Check sheet for the modelled part. Datum: model origin and axes. Units: mm. A direction names the side the tool comes from. Round coordinates to 2 decimals unless told otherwise and drop trailing zeros. Write each loop counter-clockwise with the first axis right and the second up, starting at its lowest first coordinate (ties: lowest second). Pieces come first, ordered by that corner, then holes.
from build123d import *

# Parameters (mm, degrees)
BOSS_EXTRUDE1_DEPTH = 10
BOSS_EXTRUDE2_DEPTH = 10
SKETCH3_R           = 7.5
BOSS_EXTRUDE3_DEPTH = 145
SKETCH4_R           = 2.5
BOSS_EXTRUDE4_DEPTH = 145
SKETCH6_R           = 12.5
CUT_EXTRUDE1_DEPTH  = 165
SKETCH9_R           = 7.5
CUT_EXTRUDE2_DEPTH  = 25
SKETCH11_R          = 15
BOSS_EXTRUDE6_DEPTH = 20
SKETCH12_R          = 15
BOSS_EXTRUDE7_DEPTH = 20
SKETCH13_R          = 15
CUT_EXTRUDE6_DEPTH  = 25


with BuildPart() as part:
    # Sketch1 → Boss-Extrude1 (new body)
    with BuildSketch(Plane.XY):
        with BuildLine():
            Line((-265, 35), (265, 35))
            ThreePointArc((265, 35), (300, 0), (265, -35))
            Line((265, -35), (-265, -35))
            ThreePointArc((-265, -35), (-300, 0), (-265, 35))
        make_face()
    extrude(amount=BOSS_EXTRUDE1_DEPTH)



with BuildPart() as body_2:
    # Sketch2 → Boss-Extrude2 (new body)
    with BuildSketch(Plane.XY.offset(-100)):
        with BuildLine():
            Line((-265, 35), (265, 35))
            ThreePointArc((265, 35), (300, 0), (265, -35))
            Line((265, -35), (-265, -35))
            ThreePointArc((-265, -35), (-300, 0), (-265, 35))
        make_face()
    extrude(amount=-BOSS_EXTRUDE2_DEPTH)


with BuildPart() as part_1:
    add(part.part)

    add(body_2.part)  # Boss-Extrude3 merges body 2
    # Sketch3 → Boss-Extrude3 (add)
    with BuildSketch(Plane(origin=(0, 0, -110), x_dir=(-1, 0, 0), z_dir=(0, 0, -1))):
        Circle(SKETCH3_R)
    extrude(amount=-BOSS_EXTRUDE3_DEPTH)

    # Sketch4 → Boss-Extrude4 (add)
    with BuildSketch(Plane(origin=(0, 0, -110), x_dir=(-1, 0, 0), z_dir=(0, 0, -1))):
        with Locations((200, 0)):
            Circle(SKETCH4_R)
    extrude(amount=-BOSS_EXTRUDE4_DEPTH)

    # Sketch6 → Cut-Extrude1 (cut)
    with BuildSketch(Plane(origin=(0, 0, -110), x_dir=(-1, 0, 0), z_dir=(0, 0, -1))):
        with Locations((265, 0)):
            Circle(SKETCH6_R)
    extrude(amount=-CUT_EXTRUDE1_DEPTH, mode=Mode.SUBTRACT)

    # Sketch9 → Cut-Extrude2 (cut)
    with BuildSketch(Plane.XY.offset(35)):
        with Locations((-200, 0)):
            Circle(SKETCH9_R)
    extrude(amount=-CUT_EXTRUDE2_DEPTH, mode=Mode.SUBTRACT)

    # Sketch11 → Boss-Extrude6 (add)
    with BuildSketch(Plane.XY.offset(10)):
        with Locations((265, 0)):
            Circle(SKETCH11_R)
    extrude(amount=BOSS_EXTRUDE6_DEPTH)

    # Sketch12 → Boss-Extrude7 (add)
    with BuildSketch(Plane(origin=(0, 0, -110), x_dir=(-1, 0, 0), z_dir=(0, 0, -1))):
        with Locations((-265, 0)):
            Circle(SKETCH12_R)
    extrude(amount=BOSS_EXTRUDE7_DEPTH)

    # Sketch13 → Cut-Extrude6 (cut)
    with BuildSketch(Plane.XY.offset(35)):
        Circle(SKETCH13_R)
    extrude(amount=-CUT_EXTRUDE6_DEPTH, mode=Mode.SUBTRACT)


solid = part_1.part
1. Set-up check for faces 4 (the cylindrical face through (7.493, 0.33, -50.7)), 5 (the cylindrical face through (250.693, 4.506, -119.86)), 6 (the flat face through (265, 0, -130)), 7 (the cylindrical face through (278.856, -5.745, 19.86)): record each of +Z, -Z, +X, -X, +Y, -Y from which the full face is reachable in a straight line by a thin tool's end or side.
2. Release check for a two-part mould opening along Y. For faces 1 (the flat face through (4, -35, 5)), 2 (the cylindrical face through (-276.923, 3.755, -105.07)), 3 (the cylindrical face through (-299.99, -0.77, 4.93)) record: released by +Y, released by -Y, zero draft, split by the parting line, or undercut.
3. Scan lines: line 1 along Y through (x, z) = (-265, 4); line 2 along Z through (x, y) = (96.5, 28); line 3 along X through (y, z) = (2, -66). Record each from-to range of solid material in increasing order.
4. Sectioned sample at C-C, the plane z = -44.5. Enter the section's corners in (x, y), plus the area to 3 significant figures.
5. Go/stop test with flat-tipped pins: pin 1 (1.5 mm diameter, centred on x = 9, y = 6.5, fed in from -Z); pin 2 (10 mm diameter, centred on y = 21.5, z = 2.5, fed in from +X); pin 3 (3 mm diameter, centred on x = -52.5, y = -15, fed in from +Z). Record where each tip stops, or that it passes through.
6. Sectioned sample at B-B, the plane x = -56. Enter the section's corners in (y, z).
7. Sectioned sample at D-D, the plane x = -260. Enter the section's corners in (y, z).
8. Sectioned sample at A-A, the plane y = -28. Enter the section's corners in (x, z).
Computed values:
1. face 4: none
1. face 5: -Z
1. face 6: -Z, +X, -X, +Y, -Y
1. face 7: +Z
2. face 1: released by -Y
2. face 2: undercut
2. face 3: split by the parting line
3. line 1: y = -35 to -12.5, 12.5 to 35
3. line 2: z = -110 to -100, 0 to 10
3. line 3: x = -201.5 to -198.5, -7.23 to 7.23
4. outline: circle Ø5 at (-200, 0); circle Ø15 at (0, 0)
4. area: 196 mm2
5. pin 1: stops at z = -110
5. pin 2: stops at x = 295.87
5. pin 3: stops at z = 10
6. outline: (-35, -110) - (35, -110) - (35, -100) - (-35, -100) - close; (-35, 0) - (35, 0) - (35, 10) - (-35, 10) - close
7. outline: (-35, -110) - (-11.46, -110) - (-11.46, -100) - (-35, -100) - close; (-35, 0) - (-11.46, 0) - (-11.46, 10) - (-35, 10) - close; (11.46, -110) - (35, -110) - (35, -100) - (11.46, -100) - close; (11.46, 0) - (35, 0) - (35, 10) - (11.46, 10) - close
8. outline: (-286, -110) - (286, -110) - (286, -100) - (-286, -100) - close; (-286, 0) - (286, 0) - (286, 10) - (-286, 10) - close
